Could you check a few things on this model? Use its own coordinates, in mm. A direction names the side the tool comes from. Coordinates: 2 decimals unless noted, no trailing zeros. Order: outer loops, then holes, each group sorted by start corner. A loop starts at its lowest first (then second) coordinate and runs counter-clockwise, first axis right, second up.
Autodesk Inventor part; units mm, degrees
ref_plane "YZ Plane" through (0, 0, 0) normal (1, 0, 0) x (0, 1, 0)
ref_plane "XZ Plane" through (0, 0, 0) normal (0, 1, 0) x (-1, 0, 0)
ref_plane "XY Plane" through (0, 0, 0) normal (0, 0, 1) x (1, 0, 0)
sketch "Sketch1" plane through (0, 0, 0) normal (0, 0, 1) x (1, 0, 0)
  line L0 (-1066.8, 304.8) -> (1066.8, 304.8)
  line L1 (1066.8, 304.8) -> (1066.8, -304.8)
  line L2 (1066.8, -304.8) -> (-1066.8, -304.8)
  line L3 (-1066.8, -304.8) -> (-1066.8, 304.8)
  point P0 (0, 0)
  point P1 (1066.8, 0)
  point P2 (0, 304.8)
  dimension "d0" = 2133.6
  dimension "d1" = 609.6
extrude "Extrusion1" add sketch "Sketch1" along normal mid plane 25.4
sketch "Sketch3" plane through (0, 0, 12.7) normal (0, 0, 1) x (1, 0, 0)
  line L0 (-1066.8, -304.8) -> (-1066.8, 304.8)
  line L1 (1066.8, -304.8) -> (-1066.8, -304.8)
  line L2 (-1066.8, 304.8) -> (-1041.4, 304.8)
  line L3 (-1041.4, 304.8) -> (-1041.4, -304.8)
  line L4 (-1041.4, -304.8) -> (-1066.8, -304.8)
  line L5 (-1066.8, -304.8) -> (-1066.8, 304.8)
  line L6 (1066.8, 304.8) -> (1041.4, 304.8)
  line L7 (1041.4, 304.8) -> (1041.4, -304.8)
  line L8 (1041.4, -304.8) -> (1066.8, -304.8)
  line L9 (1066.8, -304.8) -> (1066.8, 304.8)
  point P0 (0, 0)
  dimension "d18" = 25.4
  dimension "d19" = 25.4
extrude "Extrusion3" add sketch "Sketch3" along normal blind 203.2
sketch "Sketch5" plane through (0, 0, 0) normal (0, 1, 0) x (-1, 0, 0)
  line L0 (-1041.4, 12.7) -> (1041.4, 12.7)
  point P0 (0, 0)
  point P1 (787.4, 12.7)
sketch "Sketch6" plane through (0, 0, 12.7) normal (0, 0, 1) x (1, 0, 0)
  line L0 (-1041.4, 304.8) -> (-1041.4, -304.8)
  line L1 (-1041.4, 304.8) -> (-965.2, 304.8)
  line L2 (-965.2, 304.8) -> (-965.2, 177.8)
  line L3 (-965.2, 177.8) -> (-1041.4, 177.8)
  line L4 (-1041.4, 177.8) -> (-1041.4, 304.8)
  line L5 (-1041.4, -304.8) -> (-965.2, -304.8)
  line L6 (-965.2, -304.8) -> (-965.2, -177.8)
  line L7 (-965.2, -177.8) -> (-1041.4, -177.8)
  line L8 (-1041.4, -177.8) -> (-1041.4, -304.8)
  point P0 (0, 0)
  dimension "d30" = 76.2
  dimension "d31" = 127
  dimension "d32" = 127
  dimension "d33" = 76.2
extrude "Extrusion5" add sketch "Sketch6" along normal blind 203.2
mirror "Mirror1" about plane through (0, 0, 0) normal (1, 0, 0) of "Extrusion5"
fillet "Fillet1" radius 50.8 4 edges at (-965.2, 177.8, 114.3) (965.2, 177.8, 114.3) (965.2, -177.8, 114.3) (-965.2, -177.8, 114.3)
sketch "Sketch14" plane through (0, 0, -12.7) normal (0, 0, -1) x (-1, 0, 0)
  line L0 (-1066.8, 304.8) -> (1066.8, 304.8)
  line L1 (1066.8, 304.8) -> (1066.8, 330.2)
  line L2 (1066.8, 330.2) -> (-1066.8, 330.2)
  line L3 (-1066.8, 330.2) -> (-1066.8, 304.8)
  line L4 (1066.8, -304.8) -> (-1066.8, -304.8)
  line L5 (-1066.8, -304.8) -> (-1066.8, -330.2)
  line L6 (-1066.8, -330.2) -> (1066.8, -330.2)
  line L7 (1066.8, -330.2) -> (1066.8, -304.8)
  point P0 (0, 0)
  dimension "d62" = 25.4
  dimension "d63" = 25.4
extrude "Extrusion11" add sketch "Sketch14" against normal blind 228.6
sketch "Sketch15" plane through (-1066.8, 330.2, -12.7) normal (0, 1, 0) x (1, 0, 0)
  line L0 (2133.6, 0) -> (2133.6, -228.6)
  line L1 (2133.6, -228.6) -> (2133.6, -254)
  line L2 (2133.6, -254) -> (1879.6, -254)
  line L3 (1879.6, -254) -> (1371.6, -457.2)
  line L4 (1371.6, -457.2) -> (762, -457.2)
  line L5 (762, -457.2) -> (254, -254)
  line L6 (254, -254) -> (0, -254)
  line L7 (0, -254) -> (0, -228.6)
  line L8 (0, -228.6) -> (2133.6, -228.6)
  point P0 (1066.8, -12.7)
  dimension "d66" = 254
  dimension "d67" = 508
  dimension "d68" = 609.6
  dimension "d69" = 508
  dimension "d70" = 254
  dimension "d71" = 228.6
  dimension "d72" = 25.4
  dimension "d73" = 25.4
extrude "Extrusion12" add sketch "Sketch15" against normal blind 25.4
mirror "Mirror4" about plane through (0, 0, 0) normal (0, 1, 0) of "Extrusion12"
sketch "Sketch16" plane through (0, 0, -12.7) normal (0, 0, -1) x (-1, 0, 0)
  line L0 (-457.2, -177.8) -> (-457.2, -76.2)
  line L1 (-355.6, -177.8) -> (-355.6, -76.2)
  arc A0 (-355.6, -76.2) -> (-457.2, -76.2) centre (-406.4, -76.2) ccw
  arc A1 (-457.2, -177.8) -> (-355.6, -177.8) centre (-406.4, -177.8) ccw
  line L2 (-1066.8, 330.2) -> (-1066.8, -330.2)
  line L3 (-1066.8, -330.2) -> (1066.8, -330.2)
  point P0 (0, 0)
  dimension "d76" = 101.6
  dimension "d77" = 609.6
  dimension "d78" = 152.4
  dimension "d79" = 101.6
extrude "Extrusion13" cut sketch "Sketch16" against normal blind 25.4
sketch "Sketch20" plane through (0, 0, 12.7) normal (0, 0, 1) x (1, 0, 0)
  line L0 (-965.2, 304.8) -> (-1066.8, 304.8)
  line L1 (-1041.4, 304.8) -> (-749.3, 304.8)
  line L2 (-749.3, 304.8) -> (-749.3, 228.6)
  line L3 (-749.3, 228.6) -> (-1041.4, 228.6)
  line L4 (-1041.4, 228.6) -> (-1041.4, 304.8)
  line L5 (-965.2, -304.8) -> (-1028.7, -304.8)
  line L6 (-1016, -304.8) -> (-584.2, -304.8)
  line L7 (-584.2, -304.8) -> (-584.2, -228.6)
  line L8 (-584.2, -228.6) -> (-1016, -228.6)
  line L9 (-1016, -228.6) -> (-1016, -304.8)
  point P0 (0, 0)
  dimension "d106" = 431.8
extrude "Extrusion16" add sketch "Sketch20" along normal blind 101.6
mirror "Mirror5" about plane through (0, 0, 0) normal (1, 0, 0) of "Extrusion16"
sketch "Sketch21" plane through (0, 0, 12.7) normal (0, 0, 1) x (1, 0, 0)
  line L0 (812.8, 304.8) -> (304.8, 304.8)
  line L1 (681.4009, 304.8) -> (770.3009, 304.8)
  line L2 (770.3009, 304.8) -> (770.3009, 177.8)
  line L3 (770.3009, 177.8) -> (681.4009, 177.8)
  line L4 (681.4009, 177.8) -> (681.4009, 304.8)
  point P0 (0, 0)
  dimension "d91" = 127
  dimension "d92" = 88.9
extrude "Extrusion17" add sketch "Sketch21" along normal blind 101.6
sketch "Sketch22" plane through (0, 0, 12.7) normal (0, 0, 1) x (1, 0, 0)
  line L0 (-812.8, 304.8) -> (-1066.8, 304.8)
  line L1 (-812.8, -304.8) -> (-1066.8, -304.8)
  line L2 (-1041.4, 304.8) -> (-952.5, 304.8)
  line L3 (-952.5, 304.8) -> (-952.5, -304.8)
  line L4 (-952.5, -304.8) -> (-1041.4, -304.8)
  line L5 (-1041.4, -304.8) -> (-1041.4, 304.8)
  line L6 (-1041.4, -177.8) -> (-1041.4, 177.8)
  point P0 (0, 0)
  dimension "d97" = 88.9
  dimension "d98" = 0
extrude "Extrusion18" add sketch "Sketch22" along normal blind 101.6
mirror "Mirror7" about plane through (0, 0, 0) normal (1, 0, 0) of "Extrusion18"
sketch "Sketch23" plane through (-1066.8, -330.2, -12.7) normal (0, -1, 0) x (1, 0, 0)
  circle A0 centre (76.2, 76.2) radius 25.4
  line L0 (0, 0) -> (0, 254)
  line L1 (2133.6, 0) -> (0, 0)
  point P0 (1066.8, 12.7)
  dimension "d101" = 50.8
  dimension "d102" = 76.2
  dimension "d103" = 76.2
extrude "Extrusion19" cut sketch "Sketch23" against normal blind 152.4
mirror "Mirror8" about plane through (0, 0, 0) normal (1, 0, 0) of "Extrusion19"
properties part number "Cam_support"
Item 1: Suppose I cut it at D-D (y = -275.5). List the corners of the cut face in (x, z) for me.
Item 2: Thinking about a two-plate mould opening in Y: for faces 4 (the face through (-562.356, -317.678, 341.478)), 5 (the face through (584.2, -266, 63)), 6 (the face through (-965.2, 267, 164)), 7 (the face through (15, -330.2, 162)), which applies, +Y half, -Y half, draft (parallel to the pull), parting line (faces both ways), or undercut?
Item 3: Suppose I cut it at A-A (y = -110). List the corners of the cut face in (x, z) for me.
Item 4: Suppose I cut it at C-C (x = 921.5). List the corners of the cut face in (y, z) for me.
Item 5: Suppose I cut it at B-B (z = 414). List the corners of the cut face in (x, y) for me.
Item 6: Which directions (+Z, -Z, +X, -X, +Y, -Y) give clear straight access to the entire face, cutting with the end or side of a thin tool? Please do faces 1 (the face through (-991, -177.8, 64)), 2 (the face through (1049, 4, 215.9)), 3 (the face through (15, -304.8, 226)).
Item 7: For pin 1 Ø10 at (x, y) = (253, 58.5) entering from +Z, with a flat end and sliding along its axis, tell me the tip position at first contact or that it passes through.
Item 8: I need wall thicknesses on line 1 (Z direction, x = 990.6, y = -276); line 2 (Y direction, x = -794, z = 208); line 3 (Y direction, x = -733.5, z = 26). Which ranges of each line are inside material? Lowest first, please.
Geometry results:
1. outline: (-1066.8, -12.7) - (1066.8, -12.7) - (1066.8, 215.9) - (965.2, 215.9) - (965.2, 114.3) - (584.2, 114.3) - (584.2, 12.7) - (-584.2, 12.7) - (-584.2, 114.3) - (-965.2, 114.3) - (-965.2, 215.9) - (-1066.8, 215.9) - close; hole circle Ø50.8 at (-990.6, 63.5); hole circle Ø50.8 at (990.6, 63.5)
2. face 4: draft
2. face 5: undercut
2. face 6: undercut
2. face 7: -Y half
3. outline: (-1066.8, -12.7) - (355.6, -12.7) - (355.6, 12.7) - (-952.5, 12.7) - (-952.5, 114.3) - (-1041.4, 114.3) - (-1041.4, 215.9) - (-1066.8, 215.9) - close; (457.2, -12.7) - (1066.8, -12.7) - (1066.8, 215.9) - (1041.4, 215.9) - (1041.4, 114.3) - (952.5, 114.3) - (952.5, 12.7) - (457.2, 12.7) - close
4. outline: (-330.2, -12.7) - (330.2, -12.7) - (330.2, 241.3) - (304.8, 241.3) - (304.8, 114.3) - (228.6, 114.3) - (228.6, 12.7) - (-228.6, 12.7) - (-228.6, 114.3) - (-304.8, 114.3) - (-304.8, 241.3) - (-330.2, 241.3) - close
5. outline: (-381.05, -330.2) - (381.05, -330.2) - (381.05, -304.8) - (-381.05, -304.8) - close; (-381.05, 304.8) - (381.05, 304.8) - (381.05, 330.2) - (-381.05, 330.2) - close
6. face 1: -Y
6. face 2: +Z, +X, -X
6. face 3: +Z
7. pin 1: stops at z = 12.7
8. line 1: z = -12.7 to 38.1, 88.9 to 215.9
8. line 2: y = -330.2 to -304.8, 304.8 to 330.2
8. line 3: y = -330.2 to -228.6, 304.8 to 330.2
